```python
from build123d import *

# Parameters (mm, degrees)
SKETCH2_W           = 15
SKETCH2_H           = 37.5
BOSS_EXTRUDE1_DEPTH = 5
SKETCH3_W           = 15
SKETCH3_H           = 5
BOSS_EXTRUDE2_DEPTH = 20
SKETCH4_W           = 3
SKETCH4_H           = 10
BOSS_EXTRUDE3_DEPTH = 20
FILLET1_R           = 20
SKETCH6_R           = 2.65
CUT_EXTRUDE2_DEPTH  = 10
SKETCH7_R           = 2.65
CUT_EXTRUDE3_DEPTH  = 10


with BuildPart() as part:
    # Sketch2 → Boss-Extrude1 (new body)
    with BuildSketch(Plane.XY):
        with Locations((7.5, 18.75)):
            Rectangle(SKETCH2_W, SKETCH2_H)
    extrude(amount=BOSS_EXTRUDE1_DEPTH)

    # Sketch3 → Boss-Extrude2 (add)
    with BuildSketch(Plane.XY.offset(5)):
        with Locations((7.5, 2.5)):
            Rectangle(SKETCH3_W, SKETCH3_H)
    extrude(amount=BOSS_EXTRUDE2_DEPTH)

    # Sketch4 → Boss-Extrude3 (add)
    with BuildSketch(Plane(origin=(0, 0, 0), x_dir=(-1, 0, 0), z_dir=(0, 0, -1))):
        with Locations((-13.5, 32.5)):
            Rectangle(SKETCH4_W, SKETCH4_H)
        with Locations((-1.5, 32.5)):
            Rectangle(SKETCH4_W, SKETCH4_H)
    extrude(amount=BOSS_EXTRUDE3_DEPTH)

    # Fillet1
    fillet1_edges = [part.edges().sort_by_distance(p)[0] for p in [
        (1.5, 27.5, 0),
        (13.5, 27.5, 0),
    ]]
    fillet(fillet1_edges, radius=FILLET1_R - 0.0001)  # a hair under: the kernel refuses the full size

    # Sketch6 → Cut-Extrude2 (cut)
    with BuildSketch(Plane.XZ):
        with Locations(Location((7.5, 15, 0), (0, 0, 270))):
            Circle(SKETCH6_R)
    extrude(amount=-CUT_EXTRUDE2_DEPTH, mode=Mode.SUBTRACT)

    # Sketch7 → Cut-Extrude3 (cut)
    with BuildSketch(Plane(origin=(0, 0, 0), x_dir=(-1, 0, 0), z_dir=(0, 0, -1))):
        with Locations((-7.5, 15)):
            Circle(SKETCH7_R)
    extrude(amount=-CUT_EXTRUDE3_DEPTH, mode=Mode.SUBTRACT)


solid = part.part
```
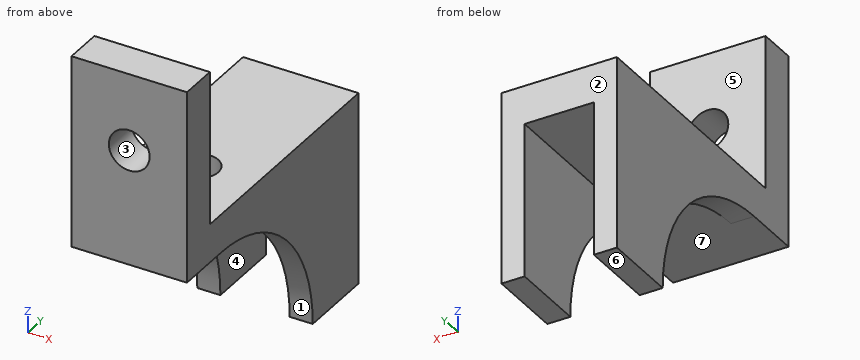
Verification items for the finished model (mm, model axes). Face numbers are marked on the shaded views. A direction names the side the tool comes from. Give positions to 0.01 mm unless a question says otherwise; leave off trailing zeros. Order: outer loops, then holes, each group sorted by start corner. A loop starts at its lowest first (then second) coordinate and runs counter-clockwise, first axis right, second up. Notation, with made-up numbers: (-33.5, 53.5) -> (-24.5, 53.5) arc R21 cw to (-24.5, 70.5) -> close; hole circle Ø10 at (64.5, 80.25). An arc over 180 degrees is marked (long way). One line per item, written item: value.
(1) Sectioned sample at A-A on z = 15. Record the cut outline in (x, y).
Final values:
outline: (0, 0) -> (4.85, 0) -> (4.85, 5) -> (0, 5) -> close; (10.15, 0) -> (15, 0) -> (15, 5) -> (10.15, 5) -> close
(2) Sectioned sample at C-C on x = 7.5. Record the cut outline in (y, z).
Final values:
outline: (0, 0) -> (12.35, 0) -> (12.35, 5) -> (5, 5) -> (5, 12.35) -> (0, 12.35) -> close; (0, 17.65) -> (5, 17.65) -> (5, 25) -> (0, 25) -> close; (17.65, 0) -> (37.5, 0) -> (37.5, 5) -> (17.65, 5) -> close
(3) Sectioned sample at B-B on y = 32. Record the cut outline in (x, z).
Final values:
outline: (0, -20) -> (3, -20) -> (3, 0) -> (12, 0) -> (12, -20) -> (15, -20) -> (15, 5) -> (0, 5) -> close
(4) Draft check along Z on the marked faces 1, 2 and 3. Enter one of: pulls with the +Z half, pulls with the -Z half, needs draft (parallel to the pull), parting line crosses it, or undercut.
Final values:
face 1: pulls with the -Z half
face 2: needs draft
face 3: undercut
(5) Gauge pin test, flat ends, axial feed: pin 1 (5 mm diameter, centred on x = 7.5, y = 15, fed in from -Z); pin 2 (7 mm diameter, centred on x = 7.5, z = 15, fed in from +Y). Record the tip position at first contact, or that the pin passes through.
Final values:
pin 1: through
pin 2: y = 5
(6) Sectioned sample at D-D on z = 2. Record the cut outline in (x, y).
Final values:
outline: (0, 0) -> (15, 0) -> (15, 37.5) -> (0, 37.5) -> close; hole circle Ø5.3 at (7.5, 15)
(7) Tool access check on the marked faces 4, 5, 6 and 7. Record the directions out of +Z, -Z, +X, -X, +Y, -Y that give a thin tool (end or side, any length) a straight path to the whole face; none if there is none.
Final values:
face 4: -Z, +Y, -Y
face 5: +Z, +X, -X, +Y
face 6: -Z, +X, -X, +Y, -Y
face 7: -Z, -Y
(8) Scan lines: line 1 along X through (y, z) = (2, 15); line 2 along Y through (x, z) = (7.5, 3.3); line 3 along X through (y, z) = (25.5, -10). Record each from-to range of solid material in increasing order. Write a range as [from, to].
Final values:
line 1: [0, 4.85], [10.15, 15]
line 2: [0, 12.35], [17.65, 37.5]
line 3: [0, 3], [12, 15]
